For this review, take the finished solid that the model builds, in its own axes (mm). A direction names the side the tool comes from. Coordinates: 2 decimals unless noted, no trailing zeros. Write each loop counter-clockwise with the first axis right and the second up, starting at its lowest first coordinate (ties: lowest second). Pieces come first, ordered by that corner, then holes.
```python
from build123d import *

# Parameters (mm, degrees)
BOSS_EXTRUDE1_DEPTH = 70
DRAFT3_ANGLE        = -34
SKETCH2_R           = 4
CUT_EXTRUDE1_DEPTH  = 70
CUT_EXTRUDE3_START  = 64.5
CUT_EXTRUDE3_DEPTH  = 1
BOSS_EXTRUDE2_DEPTH = 12
SKETCH7_R           = 1.6
CUT_EXTRUDE4_DEPTH  = 70
CUT_EXTRUDE5_START  = -6
SKETCH7_3_R         = 1.6
CUT_EXTRUDE5_DEPTH  = 70


with BuildPart() as part:
    # Sketch1 → Boss-Extrude1 (new body)
    with BuildSketch(Plane(origin=(0, 0, 0), x_dir=(1, 0, 0), z_dir=(0, 1, 0))):
        Polygon((65, 0), (130, -70), (0, -70), align=None)
    extrude(amount=BOSS_EXTRUDE1_DEPTH)

    # Draft3
    draft3_faces = [part.faces().sort_by_distance(p)[0] for p in [
        (97.5, 35, 35),
        (32.5, 35, 35),
    ]]
    draft(draft3_faces, Plane(origin=(0, 0, 0), x_dir=(0, 0, -1), z_dir=(0, -1, 0)), DRAFT3_ANGLE)

    # Sketch2 → Cut-Extrude1 (cut)
    with BuildSketch(Plane.XZ):
        with Locations((51, 31)):
            Circle(SKETCH2_R)
        with Locations((79, 31)):
            Circle(SKETCH2_R)
    extrude(amount=-CUT_EXTRUDE1_DEPTH, mode=Mode.SUBTRACT)

    # Sketch5 → Cut-Extrude3 (cut)
    with BuildSketch(Plane(origin=(0, 0, 0), x_dir=(0, 0, -1), z_dir=(1, 0, 0)).offset(CUT_EXTRUDE3_START)):
        Polygon((-14.079975623, 14.204023601), (-63.359890305, 63.918106202), (-66.397363247, 52.777769966), (-17.117448565, 3.063687364), align=None)
    extrude(amount=CUT_EXTRUDE3_DEPTH, mode=Mode.SUBTRACT)

    # Sketch6 → Boss-Extrude2 (add)
    with BuildSketch(Plane.XZ):
        Polygon((130, 70), (0, 70), (3.621428571, 66.1), (126.378571429, 66.1), align=None)
        Polygon((123.407142857, 62.9), (6.592857143, 62.9), (10.214285714, 59), (119.785714286, 59), align=None)
        Polygon((6.592857143, 62.9), (0, 62.9), (0, 59), (10.214285714, 59), align=None)
        Polygon((3.621428571, 66.1), (0, 70), (0, 66.1), align=None)
        Polygon((130, 66.1), (130, 70), (126.378571429, 66.1), align=None)
        Polygon((130, 59), (130, 62.9), (123.407142857, 62.9), (119.785714286, 59), align=None)
    extrude(amount=BOSS_EXTRUDE2_DEPTH)

    # Sketch7 → Cut-Extrude4 (cut)
    with BuildSketch(Plane(origin=(0, 0, 59), x_dir=(-1, 0, 0), z_dir=(0, 0, -1))):
        with Locations((-95, -6)):
            Circle(SKETCH7_R)
        with Locations((-123.5, -6)):
            Circle(SKETCH7_R)
        with Locations((-113.5, -6)):
            Circle(SKETCH7_R)
        with Locations((-6.5, -6)):
            Circle(SKETCH7_R)
        with Locations((-16.5, -6)):
            Circle(SKETCH7_R)
        with Locations((-35, -6)):
            Circle(SKETCH7_R)
    extrude(amount=-CUT_EXTRUDE4_DEPTH, mode=Mode.SUBTRACT)

    # Sketch7_3 → Cut-Extrude5 (cut)
    with BuildSketch(Plane(origin=(0, 0, 59), x_dir=(-1, 0, 0), z_dir=(0, 0, -1)).offset(CUT_EXTRUDE5_START)):
        Polygon((-106.5, -12), (-106.5, 0), (-119.785714286, 0), (-130, 0), (-130, -12), align=None)
        with Locations((-123.5, -6)):
            Circle(SKETCH7_3_R, mode=Mode.SUBTRACT)
        with Locations((-113.5, -6)):
            Circle(SKETCH7_3_R, mode=Mode.SUBTRACT)
        Polygon((-10.214285714, 0), (-23.5, 0), (-23.5, -12), (0, -12), (0, 0), align=None)
        with Locations((-16.5, -6)):
            Circle(SKETCH7_3_R, mode=Mode.SUBTRACT)
        with Locations((-6.5, -6)):
            Circle(SKETCH7_3_R, mode=Mode.SUBTRACT)
    extrude(amount=-CUT_EXTRUDE5_DEPTH, mode=Mode.SUBTRACT)


solid = part.part
```
1) The part is to be moulded in two halves that separate along Z. For faces 1 (the face through (4, 0, 61)), 2 (the face through (64.993, 28.269, 42.102)), 3 (the face through (45.258, 26.732, 47.759)), 4 (the face through (53.15, 8.512, 34.373)), say which applies: pulls with the +Z half, pulls with the -Z half, needs draft (parallel to the pull), parting line crosses it, or undercut.
2) Clearance check with flat-ended pins moving along their axes: P1, Ø4.5, axis at x = 5.5, z = 61.5, coming from the +Y side; P2, Ø17.5, axis at x = 45, z = 27, coming from the -Y side; P3, Ø6, axis at x = 56, y = 36.5, coming from the -Z side. State where each tip first meets the part, or that it passes through.
3) Tool access review of faces 5 (the face through (66, 0, 42)), 6 (the face through (23.5, -6, 68)), 7 (the face through (106.5, -6, 68)): name each direction out of +Z, -Z, +X, -X, +Y, -Y from which nothing blocks a thin tool from reaching the whole face with its end or side.
4) Consider section C-C (y = -6). Count the separate pieces of the cut face and the enclosed holes in it, then the cut area to 3 significant figures.
5) For L1, parallel to X at y = 9.75, z = 31; L2, parallel to Y at x = 113.5, z = 60.7; L3, parallel to X at y = 9, z = 31, list the stretches that pass through material, from the lowest coordinate up.
6) Consider section D-D (x = 69.5). Give the boundary of the cut face in (y, z).
7) Consider section A-A (z = 31). Give the boundary of the cut face in (x, y), then the cut area to 3 significant figures.
8) Consider section B-B (x = 16.5). Give the boundary of the cut face in (y, z).
Results:
1. face 1: needs draft
1. face 2: undercut
1. face 3: pulls with the -Z half
1. face 4: undercut
2. P1: stops at y = 0.74
2. P2: stops at y = 0
2. P3: stops at z = 41.48
3. face 5: -Z, +X, -X, -Y
3. face 6: +Z, -X, -Y
3. face 7: +Z, +X, -Y
4. separate pieces: 10
4. enclosed holes: 0
4. area: 731 mm2
5. L1: x = 45.19 to 47, 55 to 75, 83 to 84.81
5. L2: y = -12 to -7.6, -4.4 to 8.54
5. L3: x = 44.5 to 47, 55 to 75, 83 to 85.5
6. outline: (-12, 59) - (0, 59) - (0, 4.85) - (65.73, 70) - (-12, 70) - (-12, 66.1) - (0, 66.1) - (0, 62.9) - (-12, 62.9) - close
7. outline: (36.21, 0) - (47, 0) - (47, 11.72) - close; (55, 0) - (75, 0) - (75, 20.41) - (65.5, 30.73) - (65.5, 17.07) - (64.5, 17.07) - (64.5, 30.73) - (55, 20.41) - close; (83, 0) - (93.79, 0) - (83, 11.72) - close
7. area: 629 mm2
8. outline: (-12, 59) - (-7.6, 59) - (-7.6, 62.9) - (-12, 62.9) - close; (-4.4, 59) - (0, 59) - (0, 52.23) - (17.93, 70) - (0, 70) - (0, 62.9) - (-4.4, 62.9) - close
